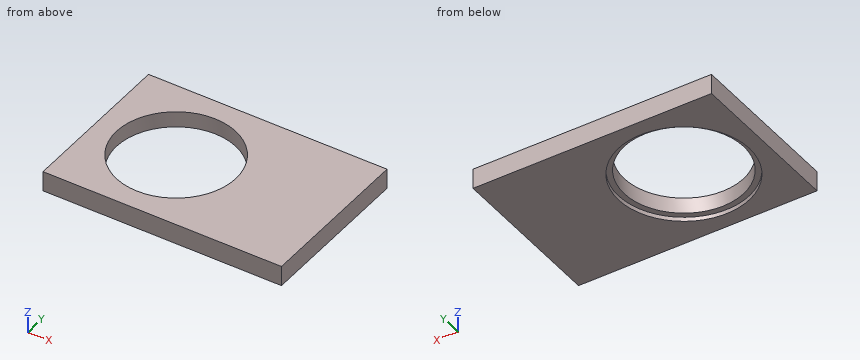
Autodesk Inventor part; units mm, degrees
ref_plane "YZ Plane" through (0, 0, 0) normal (1, 0, 0) x (0, 1, 0)
ref_plane "XZ Plane" through (0, 0, 0) normal (0, 1, 0) x (-1, 0, 0)
ref_plane "XY Plane" through (0, 0, 0) normal (0, 0, 1) x (1, 0, 0)
sketch "Sketch2" plane through (0, 0, 0) normal (0, 0, 1) x (1, 0, 0)
  circle A0 centre (0, 0) radius 18.8587
  circle A1 centre (0, 0) radius 20.6375
  dimension "d0" = 37.7174
  dimension "d1" = 41.275
extrude "Extrusion1" add sketch "Sketch2" along normal blind 5
sketch "Sketch3" plane through (0, 0, 0) normal (0, 0, -1) x (-1, 0, 0)
  circle A0 centre (0, 0) radius 20.6375
  circle A1 centre (0, 0) radius 23.1375
  dimension "d4" = 46.275
extrude "Extrusion2" add sketch "Sketch3" along normal blind 1.35 and the other way blind 5
sketch "Sketch10" plane through (0, 0, -1.35) normal (0, 0, -1) x (-1, 0, 0)
  line L0 (-25.4, -25.4) -> (25.4, -25.4)
  line L1 (25.4, -25.4) -> (25.4, 25.4)
  line L2 (25.4, 25.4) -> (-25.4, 25.4)
  line L3 (-25.4, 25.4) -> (-25.4, 0)
  line L4 (-25.4, -25.4) -> (25.4, 25.4) construction
  line L5 (25.4, -25.4) -> (-25.4, 25.4) construction
  line L6 (-25.4, 25.4) -> (-56.5021, 25.4)
  line L7 (-50, -25.4) -> (-25.4, -25.4)
  line L8 (-25.4, 0) -> (-25.4, 25.4)
  line L9 (0, 0) -> (-50, 0)
  line L10 (-50, 0) -> (-50, 25.4)
  line L11 (-50, 0) -> (-50, -25.4)
  circle A0 centre (0, 0) radius 23.1375
  dimension "d46" = 50.8
  dimension "d47" = 50.8
  dimension "d48" = 50
extrude "Extrusion9" add sketch "Sketch10" against normal blind 6.35
properties part number "3102_Biax_Coil_Mounting_Bracket_MPSv2_v1" material "Aluminum 6061"
CAD build for the part. Positions are in the model's coordinates, mm. Coordinates: 2 decimals unless noted, no trailing zeros. Write each loop counter-clockwise with the first axis right and the second up, starting at its lowest first coordinate (ties: lowest second). Pieces come first, ordered by that corner, then holes. Notation, with made-up numbers: (81, 50) -> (118, 50) arc R14 ccw to (118, 69) -> close; hole circle Ø10 at (-5.75, 17.5). An arc over 180 degrees is marked (long way). Use CSV: the item, a comma, the result in double quotes. Start each with the question number.
Item 1: Band-saw the part on B-B, the plane x = 0. Write the cut outline in (y, z).
Item 2: Wall check: probe 1 along Y at (x, z) = (0, 2.7); probe 2 along Y at (x, z) = (0, -0.45); probe 3 along Z at (x, y) = (-4.5, -19). Give the ranges that are in metal, low to high.
Item 3: Drop a flat-ended pin along its axis: P1, Ø20.5, axis at x = -4.5, y = 5, coming from the -Z side. Give the stop position or say it passes through.
Item 4: Band-saw the part on C-C, the plane z = 2.5. Write the cut outline in (x, y).
Item 5: Band-saw the part on A-A, the plane y = 0. Write the cut outline in (x, z).
Response values:
1,outline,"(-25.4, -1.35) -> (-20.64, -1.35) -> (-20.64, 0) -> (-18.86, 0) -> (-18.86, 5) -> (-25.4, 5) -> close; (18.86, 0) -> (20.64, 0) -> (20.64, -1.35) -> (25.4, -1.35) -> (25.4, 5) -> (18.86, 5) -> close"
2,probe 1,"y = -25.4 to -18.86, 18.86 to 25.4"
2,probe 2,"y = -25.4 to -20.64, 20.64 to 25.4"
2,probe 3,"z = 0 to 5"
3,P1,"passes through"
4,outline,"(-25.4, -25.4) -> (50, -25.4) -> (50, 25.4) -> (-25.4, 25.4) -> close; hole circle Ø37.72 at (0, 0)"
5,outline,"(-25.4, -1.35) -> (-20.64, -1.35) -> (-20.64, 0) -> (-18.86, 0) -> (-18.86, 5) -> (-25.4, 5) -> close; (18.86, 0) -> (20.64, 0) -> (20.64, -1.35) -> (50, -1.35) -> (50, 5) -> (18.86, 5) -> close"
